Part model, mm, in its own coordinate system. A direction names the side the tool comes from. Coordinates: 2 decimals unless noted, no trailing zeros. Loops run counter-clockwise (first coordinate to the right, second up) from the corner with the lowest first, then second, coordinate; pieces in that order, holes last. Notation, with made-up numbers: (72, 23.5) - (131, 23.5) arc R18 cw to (131, 52.5) - close; hole circle Ø11 at (56.5, 56.5). An arc over 180 degrees is marked (long way). Use a Markdown table: item, result. Add a question column.
1. Wall check: probe 1 along Z at (x, y) = (37, 26); probe 2 along X at (y, z) = (24, 121). Give the ranges that are in metal, low to high. Write a range as [from, to].
2. Drop flat-ended pins along their axis: pin 1 (4 mm diameter, centred on x = 43.14, y = 25.89, fed in from +Z); pin 2 (1.5 mm diameter, centred on x = 36.83, y = 16.55, fed in from +Z). Give the stop position or say it passes through.
3. Band-saw the part on C-C, the plane y = 29.5. Give the cut face in (x, z), plus the area to 3 significant figures.
4. Band-saw the part on B-B, the plane z = 120.5. Give the cut face in (x, y).
5. 3-axis set-ups, long thin cutter, end or side, ignore diameter. For faces 3 (the flat face through (68, 21, 118.451)), 4 (the flat face through (70.744, 21, 124)), 5 (the flat face through (44, 12, 131)): which of +Z, -Z, +X, -X, +Y, -Y reach the whole face in a straight line?
6. Band-saw the part on A-A, the plane x = 66.5. Give the cut face in (y, z).
7. Pull direction Y, two halves, no side cores. Call faces 1 (the cylindrical face through (35.58, 16.6, 133.03)), 2 (the flat face through (55, 21, 136)): pulls with the +Y half, pulls with the -Y half, needs draft (parallel to the pull), parting line crosses it, or undercut.
from build123d import *

# Parameters (mm, degrees)
SKETCH057_W     = 55
SKETCH057_H     = 39.5
PAD028_DEPTH    = 23
SKETCH058_W     = 10
SKETCH058_H     = 3
POCKET011_DEPTH = 5
SKETCH059_R     = 11.5
POCKET012_DEPTH = 1
SKETCH060_R     = 1.25
POCKET013_DEPTH = 4
SKETCH061_R     = 1.5
SKETCH061_R_2   = 1.15
POCKET014_DEPTH = 5


with BuildPart() as part:
    # Sketch057 → Pad028 (new body)
    with BuildSketch(Plane.XY):
        with Locations((8.244135, 0.838188)):
            Rectangle(SKETCH057_W, SKETCH057_H)
    extrude(amount=PAD028_DEPTH)

    # Sketch058 (on Face3 of Pad028) → Pocket011 (cut)
    with BuildSketch(Plane.YZ.offset(35.744135)):
        with Locations((0.852094, 6.951404)):
            Rectangle(SKETCH058_W, SKETCH058_H)
    extrude(amount=-POCKET011_DEPTH, mode=Mode.SUBTRACT)

    # Sketch059 (on Face5 of Pocket011) → Pocket012 (cut)
    with BuildSketch(Plane.XY.offset(23)):
        with Locations((8.142509, 0.739769)):
            Circle(SKETCH059_R)
    extrude(amount=-POCKET012_DEPTH, mode=Mode.SUBTRACT)

    # Sketch060 (on Face12 of Pocket012) → Pocket013 (cut)
    with BuildSketch(Plane.XY.offset(22)):
        with Locations((2.355179, 5.854206)):
            Circle(SKETCH060_R)
        with Locations((8.142534, 5.893073)):
            Circle(SKETCH060_R)
        with Locations((13.992255, 6.068044)):
            Circle(SKETCH060_R)
        with Locations((0.067154, 1.278166)):
            Circle(SKETCH060_R)
        with Locations((5.046978, 1.412754)):
            Circle(SKETCH060_R)
        with Locations((10.295966, 1.412754)):
            Circle(SKETCH060_R)
        with Locations((1.82863, -3.450897)):
            Circle(SKETCH060_R)
        with Locations((7.604173, -4.105418)):
            Circle(SKETCH060_R)
        with Locations((12.987754, -3.836237)):
            Circle(SKETCH060_R)
        with Locations((8.547656, -7.839936)):
            Circle(SKETCH060_R)
        with Locations((8.00794, 10.161071)):
            Circle(SKETCH060_R)
        with Locations((16.083309, 1.951109)):
            Circle(SKETCH060_R)
    extrude(amount=-POCKET013_DEPTH, mode=Mode.SUBTRACT)

    # Sketch061 (on Face1 of Pocket013) → Pocket014 (cut)
    with BuildSketch(Plane(origin=(-19.255865, 0, 0), x_dir=(0, -1, 0), z_dir=(-1, 0, 0))):
        with Locations((-14.325696, 5.317757)):
            Circle(SKETCH061_R)
        with Locations((-14.325696, 5.317757)):
            Circle(SKETCH061_R_2, mode=Mode.SUBTRACT)
    extrude(amount=-POCKET014_DEPTH, mode=Mode.SUBTRACT)


with BuildPart() as part_1:
    # Body009 placement: moved
    add(part.part.moved(Location((35, 20, 113))))


solid = part_1.part
Geometry check:
| question | item | result |
|---|---|---|
| 1 | probe 1 | z = [113, 131] |
| 1 | probe 2 | x = [15.74, 65.74] |
| 2 | pin 1 | stops at z = 135 |
| 2 | pin 2 | stops at z = 131 |
| 3 | outline | (15.74, 113) - (70.74, 113) - (70.74, 136) - (50.59, 136) - (50.59, 135) - (44.07, 135) - (44.07, 131) - (41.95, 131) - (41.95, 135) - (35.69, 135) - (35.69, 136) - (15.74, 136) - close |
| 3 | area | 1,240 mm^2 |
| 4 | outline | (15.74, 1.09) - (70.74, 1.09) - (70.74, 15.85) - (65.74, 15.85) - (65.74, 25.85) - (70.74, 25.85) - (70.74, 40.59) - (15.74, 40.59) - close |
| 5 | face 3 | +X |
| 5 | face 4 | +Z, -Z, +X, +Y, -Y |
| 5 | face 5 | +Z |
| 6 | outline | (1.09, 113) - (40.59, 113) - (40.59, 136) - (1.09, 136) - close; hole (15.85, 118.45) - (25.85, 118.45) - (25.85, 121.45) - (15.85, 121.45) - close |
| 7 | face 1 | undercut |
| 7 | face 2 | needs draft |
